Here's how the part is built. I have some questions about the finished solid (model axes, mm). A direction names the side the tool comes from. Give positions to 0.01 mm unless a question says otherwise; leave off trailing zeros. Write each loop counter-clockwise with the first axis right and the second up, starting at its lowest first coordinate (ties: lowest second). Pieces come first, ordered by that corner, then holes. Notation, with made-up numbers: M 59,-16 L 67,-16 A16 cw 67,13 Z; hole C 62.25,39.25 d3. An arc over 180 degrees is marked long. Answer as CSV lines item,"result". Start each with the question number.
Q1. Suppose I cut it at C-C (y = -37.5). Write out the boundary of the cut face in (x, z), then the cut area to 3 significant figures.
Q2. If I drill on line 1 along Y through (x, z) = (0, 2.2); line 2 along Z through (x, y) = (-21.35, -37.5); line 3 along Z through (x, y) = (-18, 0), over which ranges is the centre line in solid material (lowest first)?
Q3. Thinking about a two-plate mould opening in X: for faces 1 (the cylindrical face through (21.787, -51.748, 2.521)), 2 (the cylindrical face through (-19.97, -36.16, 24.61)), 3 (the cylindrical face through (0.54, -35.06, 2.53)), which applies, +X half, -X half, draft (parallel to the pull), parting line (faces both ways), or undercut?
Q4. For pin 1 (6.5 mm diameter, centred on x = 0, z = 60, fed in from -Y); pin 2 (8 mm diameter, centred on y = -36.5, z = 30.5, fed in from +X); pin 3 (8 mm diameter, centred on x = 16.5, y = -2.5, fed in from +Z), each with a flat end and sliding along its axis, tell me the tip position at first contact or that it passes through.
Q5. Suppose I cut it at A-A (z = 60). Write out the boundary of the cut face in (x, y), then the cut area to 3 significant figures.
Q6. Suppose I cut it at D-D (z = 22.5). Write out the boundary of the cut face in (x, y), then the cut area to 3 significant figures.
Q7. Suppose I cut it at B-B (x = 0). Write out the boundary of the cut face in (y, z).
Q8. On a 3-axis mill with a long thin cutter (end or side, diameter ignored), from which of +Z, -Z, +X, -X, +Y, -Y can I reach the whole of each face in a straight line? I mean faces 4 (the flat face through (-20, -37, 45)), 5 (the flat face through (2, -17, 5)), 6 (the flat face through (0, -14, 0)). Say none if no direction works.
```python
from build123d import *

# Parameters (mm, degrees)
F0_W          = 45
F0_H          = 45
F1_DEPTH      = 45
F2_T          = -5
F3_DEPTH      = 30
F4_DEPTH      = 30
F10_D         = 5
F10_2_D       = 5
F10_ON_F6_D   = 5
F10_ON_F7_D   = 5
F10_ON_F9_D   = 5
F10_ON_F9_2_D = 5
F10_ON_F5_D   = 5
F12_R         = 2.5
F13_R         = 1


with BuildPart() as f1:
    # F0 (on Top) → F1 (new body)
    with BuildSketch(Plane.XY):
        Rectangle(F0_W, F0_H)
    extrude(amount=F1_DEPTH)

    # F2
    f2_openings = [f1.faces().sort_by_distance(p)[0] for p in [
        (0, 0, 45),
        (22.5, 0, 22.5),
        (0, -22.5, 22.5),
    ]]
    offset(amount=F2_T, openings=f2_openings)


with BuildPart() as f3:
    # F3 (new): a face of the model
    f3_faces = [f1.part.faces().sort_by_distance(p)[0] for p in [
        (21.8636038969, -22.5, 2.5),
    ]]
    extrude(f3_faces, amount=F3_DEPTH)

    # F10 on F9#2 (through all)
    with Locations(Plane(origin=(0, 0, 0), x_dir=(1, 0, 0), z_dir=(0, 0, -1))):
        with Locations((0, 0), (0, 37.5)):
            Hole(F10_ON_F9_2_D / 2)

    # F10 on F5 (through all)
    with Locations(Plane(origin=(-22.5, 0, 0), x_dir=(0, -1, 0), z_dir=(-1, 0, 0))):
        with Locations((37.5, 22.5)):
            Hole(F10_ON_F5_D / 2)


with BuildPart() as f4:
    # F4 (new): a face of the model
    f4_faces = [f1.part.faces().sort_by_distance(p)[0] for p in [
        (0, 21.8636038969, 45),
    ]]
    extrude(f4_faces, amount=F4_DEPTH)

    # F10#2 (through all)
    with Locations(Plane(origin=(0, 22.5, 0), x_dir=(-1, 0, 0), z_dir=(0, 1, 0))):
        with Locations((0, 60), (0, 22.5)):
            Hole(F10_2_D / 2)

    # F10 on F6 (through all)
    with Locations(Plane(origin=(-22.5, 0, 0), x_dir=(0, -1, 0), z_dir=(-1, 0, 0))):
        with Locations((0, 60)):
            Hole(F10_ON_F6_D / 2)


with BuildPart() as f1_1:
    add(f1.part)

    # F10 (through all)
    with Locations(Plane(origin=(0, 22.5, 0), x_dir=(-1, 0, 0), z_dir=(0, 1, 0))):
        with Locations((0, 60), (0, 22.5)):
            Hole(F10_D / 2)

    # F10 on F7 (through all)
    with Locations(Plane(origin=(-22.5, 0, 0), x_dir=(0, -1, 0), z_dir=(-1, 0, 0))):
        with Locations((0, 22.5)):
            Hole(F10_ON_F7_D / 2)

    # F10 on F9 (through all)
    with Locations(Plane(origin=(0, 0, 0), x_dir=(1, 0, 0), z_dir=(0, 0, -1))):
        with Locations((0, 0), (0, 37.5)):
            Hole(F10_ON_F9_D / 2)

    # F11: union F3, F4
    add(f3.part)
    add(f4.part)

    # F12
    f12_edges = [f1_1.edges().sort_by_distance(p)[0] for p in [
        (-20, -22.5, 45),
        (-20, -22.5, 75),
        (-20, -52.5, 45),
        (22.5, 20, 75),
        (22.5, -52.5, 2.5),
    ]]
    fillet(f12_edges, radius=F12_R)

    # F13
    f13_edges = [f1_1.edges().sort_by_distance(p)[0] for p in [
        (1.25, 17.5, 75),
        (-17.5, -1.25, 75),
        (1.25, -52.5, 5),
        (-1.25, 22.5, 75),
        (22.5, -13.75, 0),
        (0, 22.5, 0),
        (-22.5, 1.25, 75),
        (-22.5, 22.5, 37.5),
        (-22.5, -15, 0),
    ]]
    fillet(f13_edges, radius=F13_R)


solid = f1_1.part
```
Resolved:
1,outline,"M -22.5,1 A1 ccw -21.5,0 L -2.5,0 L -2.5,5 L -17.5,5 L -17.5,20 L -22.5,20 Z; M -22.5,25 L -17.5,25 L -17.5,44 A1 ccw -18.5,45 L -21.5,45 A1 ccw -22.5,44 Z; M 2.5,0 L 21.5,0 A1 ccw 22.5,1 L 22.5,4 A1 ccw 21.5,5 L 2.5,5 Z"
1,area,"374 mm^2"
2,line 1,"-52.5 to -40, -35 to -2.5, 2.5 to 22.5"
2,line 2,"0 to 20, 25 to 45"
2,line 3,"0 to 20, 25 to 57.5, 62.5 to 74.87"
3,face 1,"+X half"
3,face 2,"draft"
3,face 3,"undercut"
4,pin 1,"y = 17.5"
4,pin 2,"x = -17.5"
4,pin 3,"z = 5"
5,outline,"M -22.5,-21.5 A1 ccw -21.5,-22.5 L -18.5,-22.5 A1 ccw -17.5,-21.5 L -17.5,-2.5 L -22.5,-2.5 Z; M -22.5,2.5 L -17.5,2.5 L -17.5,17.5 L -2.5,17.5 L -2.5,22.5 L -21.5,22.5 A1 ccw -22.5,21.5 Z; M 2.5,17.5 L 21.5,17.5 A1 ccw 22.5,18.5 L 22.5,21.5 A1 ccw 21.5,22.5 L 2.5,22.5 Z"
5,area,"374 mm^2"
6,outline,"M -22.5,-51.5 A1 ccw -21.5,-52.5 L -18.5,-52.5 A1 ccw -17.5,-51.5 L -17.5,-40 L -22.5,-40 Z; M -22.5,-35 L -17.5,-35 L -17.5,-2.5 L -22.5,-2.5 Z; M -22.5,2.5 L -17.5,2.5 L -17.5,17.5 L -2.5,17.5 L -2.5,22.5 L -21.5,22.5 A1 ccw -22.5,21.5 Z; M 2.5,17.5 L 21.5,17.5 A1 ccw 22.5,18.5 L 22.5,21.5 A1 ccw 21.5,22.5 L 2.5,22.5 Z"
6,area,"499 mm^2"
7,outline,"M -52.5,1 A1 ccw -51.5,0 L -40,0 L -40,5 L -51.5,5 A1 ccw -52.5,4 Z; M -35,0 L -2.5,0 L -2.5,5 L -35,5 Z; M 2.5,0 L 21.5,0 A1 ccw 22.5,1 L 22.5,20 L 17.5,20 L 17.5,5 L 2.5,5 Z; M 17.5,25 L 22.5,25 L 22.5,57.5 L 17.5,57.5 Z; M 17.5,62.5 L 22.5,62.5 L 22.5,74 A1 ccw 21.5,75 L 18.5,75 A1 ccw 17.5,74 Z"
8,face 4,"+Z, +X, -X, -Y"
8,face 5,"+Z, +X, -Y"
8,face 6,"-Z, +X, -X, +Y, -Y"
